Can you work these out from the model? Positions are in its coordinate system, mm. Face numbers are marked on the shaded views. A direction names the side the tool comes from. Give positions to 0.01 mm unless a question says otherwise; leave off trailing zeros. Write each loop counter-clockwise with the first axis right and the second up, starting at its lowest first coordinate (ties: lowest second). Pieces come first, ordered by that corner, then holes.
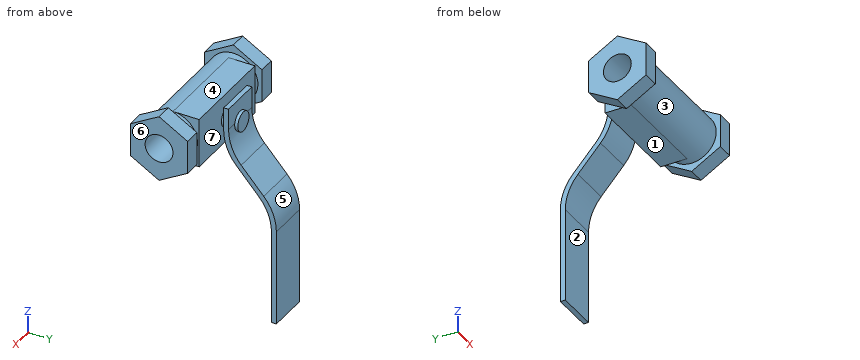
from build123d import *

# Parameters (mm, degrees)
SKETCH1_R               = 15
SKETCH1_R_2             = 5
EXTRUDE_THIN1_DEPTH     = 45
SKETCH2_W               = 60
SKETCH2_H               = 30
BOSS_EXTRUDE1_DEPTH     = 16
SKETCH3_R               = 6
BOSS_EXTRUDE2_DEPTH     = 10
EXTRUDE_THIN2_DEPTH     = 12.5
FILLET1_R               = 30
BOSS_EXTRUDE3_DEPTH     = 10
CUT_EXTRUDE1_DEPTH      = 133.543633763
CUT_EXTRUDE1_DEPTH_BACK = 133.543633763
SKETCH6_R               = 8.5


with BuildPart() as part:
    # Sketch1 → Extrude-Thin1 (new, symmetric)
    with BuildSketch(Plane(origin=(0, 0, 0), x_dir=(0, 0, -1), z_dir=(1, 0, 0))):
        Circle(SKETCH1_R)
        Circle(SKETCH1_R_2, mode=Mode.SUBTRACT)
    extrude(amount=EXTRUDE_THIN1_DEPTH, both=True)

    # Sketch2 → Boss-Extrude1 (add)
    with BuildSketch(Plane(origin=(0, 0, 0), x_dir=(1, 0, 0), z_dir=(0, 1, 0))):
        Rectangle(SKETCH2_W, SKETCH2_H)
    extrude(amount=BOSS_EXTRUDE1_DEPTH)

    # Sketch3 → Boss-Extrude2 (add)
    with BuildSketch(Plane(origin=(0, 16, 0), x_dir=(1, 0, 0), z_dir=(0, 1, 0))):
        with Locations(Location((0, 0, 0), (0, 0, 270))):
            Circle(SKETCH3_R)
    extrude(amount=BOSS_EXTRUDE2_DEPTH)

    # Sketch4 → Extrude-Thin2 (add, symmetric)
    with BuildSketch(Plane(origin=(0, 0, 0), x_dir=(0, 0, -1), z_dir=(1, 0, 0))):
        Polygon((-14.175668382, 24.036944014), (10.301514998, 24.036944014), (42.733043078, 53.23603901), (112.733043078, 53.23603901), (112.733043078, 50.23603901), (43.884565313, 50.23603901), (11.453037232, 21.036944014), (-14.175668382, 21.036944014), align=None)
    extrude(amount=EXTRUDE_THIN2_DEPTH, both=True)

    # Fillet1
    # the kernel refuses this fillet: 30 mm, written as the material it adds along each edge
    with BuildSketch(Plane(origin=(12.5, 50.23603901, -43.884565313), x_dir=(0, -0.6691004351822666, 0.7431719906178524), z_dir=(-1, 0, 0))) as fillet1_piece_1:
        with BuildLine():
            CenterArc((FILLET1_R * 0.383840744794, -FILLET1_R), FILLET1_R, 90, 41.997673873)
            Line((-FILLET1_R * 0.285259690389, -FILLET1_R * 0.256828009382), (0, 0))
            Line((0, 0), (FILLET1_R * 0.383840744794, 0))
        make_face()
    extrude(amount=25)
    with BuildSketch(Plane(origin=(12.5, 24.036944014, -10.301514998), x_dir=(0, 0, 1), z_dir=(-1, 0, 0))) as fillet1_piece_2:
        with BuildLine():
            CenterArc((FILLET1_R * 0.383840744794, FILLET1_R), FILLET1_R, 228.002326127, 41.997673873)
            Line((-FILLET1_R * 0.285259690389, FILLET1_R * 0.256828009382), (0, 0))
            Line((0, 0), (FILLET1_R * 0.383840744794, 0))
        make_face()
    extrude(amount=25)
    # the kernel refuses this fillet: 30 mm, written as the material it takes off along each edge
    with BuildSketch(Plane(origin=(41.28805586, 53.23603901, -42.733043078), x_dir=(0, -0.6691004351822663, 0.7431719906178528), z_dir=(-1, 0, 0))) as fillet1_2_piece_1:
        with BuildLine():
            CenterArc((FILLET1_R * 0.383840744794, -FILLET1_R), FILLET1_R, 90, 41.997673873)
            Line((-FILLET1_R * 0.285259690389, -FILLET1_R * 0.256828009382), (0, 0))
            Line((0, 0), (FILLET1_R * 0.383840744794, 0))
        make_face()
    extrude(amount=82.576111719, mode=Mode.SUBTRACT)
    with BuildSketch(Plane(origin=(-41.28805586, 21.036944014, -11.453037232), x_dir=(0, 0, 1), z_dir=(1, 0, 0))) as fillet1_2_piece_2_section:
        with BuildLine():
            CenterArc((FILLET1_R * 0.383840744794, -FILLET1_R), FILLET1_R, 90, 41.997673873)
            Line((-FILLET1_R * 0.285259690389, -FILLET1_R * 0.256828009382), (0, 0))
            Line((0, 0), (FILLET1_R * 0.383840744794, 0))
        make_face()
    fillet1_2_piece_2 = extrude(amount=82.576111719, mode=Mode.PRIVATE)
    fillet1_2_piece_2 = fillet1_2_piece_2 - Plane(origin=(0, 22.678661346, 0), x_dir=(0, 0, 1), z_dir=(0, -1, 0)) * Cylinder(6, 212, mode=Mode.PRIVATE)
    add(fillet1_2_piece_2, mode=Mode.SUBTRACT)

    # Sketch5 → Boss-Extrude3 (add)
    with BuildSketch(Plane(origin=(45, 0, 0), x_dir=(0, 0, -1), z_dir=(1, 0, 0))):
        Polygon((-20.207259422, 0), (-10.103629711, -17.5), (10.103629711, -17.5), (20.207259422, 0), (10.103629711, 17.5), (-10.103629711, 17.5), align=None)
    boss_extrude3 = extrude(amount=-BOSS_EXTRUDE3_DEPTH)

    # Mirror1: Boss-Extrude3 across plane
    add(boss_extrude3.mirror(Plane(origin=(0, 0, 0), x_dir=(0, 0, 1), z_dir=(1, 0, 0))))

    # Sketch6 → Cut-Extrude1 (cut, two sides: drawn at the far end of the back side and taken through both)
    with BuildSketch(Plane(origin=(0, 0, 0), x_dir=(0, 0, -1), z_dir=(1, 0, 0)).offset(-CUT_EXTRUDE1_DEPTH_BACK)):
        Circle(SKETCH6_R)
    extrude(amount=CUT_EXTRUDE1_DEPTH + CUT_EXTRUDE1_DEPTH_BACK, mode=Mode.SUBTRACT)


solid = part.part
(1) If we mould it in two halves opening along Y, with no side actions, what happens to the marked faces 5, 6 and 7? For each: +Y half, -Y half, draft (parallel to the pull), parting line (faces both ways), or undercut.
Returned:
face 5: +Y half
face 6: draft
face 7: undercut
(2) Will these pins go through, and if not, where does the flat tip stop? P1, Ø22, axis at y = 0, z = 0, coming from the -X side; P2, Ø0.9, axis at x = 5.5, y = 22.5, coming from the +Z side; P3, Ø17.5, axis at x = -12.5, y = 9, coming from the -Z side; P4, Ø14.5, axis at x = 6, z = 8, coming from the +Y side.
Returned:
P1: stops at x = -45
P2: stops at z = 14.18
P3: stops at z = -15
P4: stops at y = 26
(3) If I drill on L1, parallel to Y at x = -9, z = 0; L2, parallel to Z at x = -24, y = 0; L3, parallel to Y at x = -4.5, z = 0, over which ranges is the centre line in solid material (lowest first)?
Returned:
L1: y = -15 to -8.5, 8.5 to 16, 21.04 to 24.06
L2: z = -15 to -8.5, 8.5 to 15
L3: y = -15 to -8.5, 8.5 to 26
(4) For the marked faces 1, 2, 3 and 4, which set-ups out of +Z, -Z, +X, -X, +Y, -Y let a thin tool reach every point of the face, with its end or its side?
Returned:
face 1: -Z, -Y
face 2: -Z, +X, -X, -Y
face 3: none
face 4: +Z, +Y, -Y
(5) Imagine slicing it at A-A, the plane x = -36.5. Write out the boundary of the cut face in (y, z).
Returned:
outline: (-17.5, -10.1) - (0, -20.21) - (17.5, -10.1) - (17.5, 10.1) - (0, 20.21) - (-17.5, 10.1) - close; hole circle Ø17 at (0, 0)
(6) Imagine slicing it at D-D, the plane x = 17. Write out the boundary of the cut face in (y, z).
Returned:
outline: (0, -15) - (16, -15) - (16, 15) - (0, 15) arc R15 ccw to start; hole circle Ø17 at (0, 0)
(7) Imagine slicing it at B-B, the plane z = -81.5. Write out the boundary of the cut face in (x, y).
Returned:
outline: (-12.5, 50.24) - (12.5, 50.24) - (12.5, 53.24) - (-12.5, 53.24) - close
(8) Imagine slicing it at C-C, the plane y = 11. Write out the boundary of the cut face in (x, z).
Returned:
outline: (-45, -13.86) - (-35, -13.86) - (-35, -10.2) - (-30, -10.2) - (-30, -15) - (30, -15) - (30, -10.2) - (35, -10.2) - (35, -13.86) - (45, -13.86) - (45, 13.86) - (35, 13.86) - (35, 10.2) - (30, 10.2) - (30, 15) - (-30, 15) - (-30, 10.2) - (-35, 10.2) - (-35, 13.86) - (-45, 13.86) - close
